The model under review builds one solid part; all positions refer to its coordinate system, in mm. A direction names the side the tool comes from. Give positions to 0.01 mm unless a question says otherwise; leave off trailing zeros. Loops run counter-clockwise (first coordinate to the right, second up) from the corner with the lowest first, then second, coordinate; pieces in that order, holes last. Notation, with made-up numbers: M 12.25,34 L 51.25,34 A24 cw 51.25,45 Z; hole C 72,56.5 d4. An arc over 180 degrees is marked long. Return JSON: item names as keys, results as strings. Group by question number.
```python
from build123d import *

# Parameters (mm, degrees)
LINEAR_AUSTRAGEN1_DEPTH      = 4.035
LINEAR_AUSTRAGEN1_DEPTH_BACK = 4.035


with BuildPart() as part:
    # Skizze1 → Rotation1 (revolve)
    with BuildSketch(Plane.XY, mode=Mode.PRIVATE) as rotation1_sk:
        Polygon((0, 13.2), (3.45, 13.2), (4.35078189, 11.6398), (6, 11.6398), (6.9, 11.220123108), (6.9, -11.742857143), (6.21, -11.742857143), (6.21, -13.7), (4.864, -13.7), (4.864, -18.019), (4.283, -18.6), (3.648, -18.6), (3.648, -8.872), (0, -8.872), align=None)
    revolve(rotation1_sk.sketch.rotate(Axis((0, -18.6, 0), (0, 1, 0)), 270), axis=Axis((0, -18.6, 0), (0, 1, 0)))

    # Skizze2 → Linear austragen1 (cut, two sides: drawn at the far end of the back side and taken through both)
    with BuildSketch(Plane(origin=(0, 11.6398, 0), x_dir=(-1, 0, 0), z_dir=(0, 1, 0)).offset(-LINEAR_AUSTRAGEN1_DEPTH_BACK)):
        Polygon((7.8, -4.5033321), (7.8, 4.5033321), (0, 9.006664199), (-7.8, 4.5033321), (-7.8, -4.5033321), (-0.05, -8.977796686), (-0.05, -6.899335717), (-6, -3.464101615), (-6, 3.464101615), (0, 6.92820323), (6, 3.464101615), (6, -3.464101615), (0, -6.92820323), (0, -9.006664199), align=None)
    extrude(amount=LINEAR_AUSTRAGEN1_DEPTH + LINEAR_AUSTRAGEN1_DEPTH_BACK, mode=Mode.SUBTRACT)

    # Skizze3 → Rotation2 (revolve)
    with BuildSketch(Plane.XY, mode=Mode.PRIVATE) as rotation2_sk:
        Polygon((0, 0), (0, 6.21), (8.832, 6.21), (10.902, 6.25), (18.761, 6.25), (18.761, 5), (21.074, 5), (21.074, 4.166666667), (23.387, 4.166666667), (23.387, 6.25), (25.186, 6.25), (25.7, 4.331725885), (25.7, 3), (7.7, 3), (7.7, 0), align=None)
    revolve(rotation2_sk.sketch.rotate(Axis((25.7, 0, 0), (-1, 0, 0)), 270), axis=Axis((25.7, 0, 0), (-1, 0, 0)))


solid = part.part
```
(1) For faces 1 (the flat face through (3, 7.605, 6)), 2 (the flat face through (3.2, 7.605, -5.4)), 3 (the cylindrical face through (16.57, 0.9, 2.86)), 4 (the flat face through (-6, 10, 0)), list the 3-axis set-ups (+Z, -Z, +X, -X, +Y, -Y) from which the entire face can be reached by the end or side of a thin tool; tool diameter is ignored.
(2) Mouldability with a two-part tool opening along X and no side actions: class faces 5 (the cylindrical face through (1.46, -15.89, 4.64)), 6 (the flat face through (-2, -13.7, -5)), 7 (the cylindrical face through (6.608, 0.273, -6.204)) as released by +X, released by -X, zero draft, split by the parting line, or undercut.
(3) For probe 1 along X at (y, z) = (-14.5, 0); probe 2 along Y at (x, z) = (20, 0); probe 3 along Y at (x, z) = (15, 0), list the stretches that pass through material, from the lowest coordinate up.
(4) Add section C-C (x = 9.5). Write out the cut boundary in (y, z).
(5) For pin 1 (1 mm diameter, centred on y = -8, z = 1.5, fed in from -X); pin 2 (4 mm diameter, centred on x = 6.5, y = 6.5, fed in from -Z); pin 3 (3.5 mm diameter, centred on x = -2, z = 6, fed in from +Y); pin 4 (5 mm diameter, centred on y = 1, z = 0, fed in from +X), all flat-tipped, find the tip position at first contact; note any pin that passes through.
(6) Add section B-B (y = -13). Write out the cut boundary in (x, z).
Verdict:
{
 "1": {"face 1": "+Z, +X, +Y", "face 2": "-Z, +X, +Y", "face 3": "+X", "face 4": "+Z, -Z, -X, +Y"},
 "2": {"face 5": "split by the parting line", "face 6": "zero draft", "face 7": "undercut"},
 "3": {"probe 1": "x = -4.86 to -3.65, 3.65 to 4.86", "probe 2": "y = -5 to -3, 3 to 5", "probe 3": "y = -6.25 to -3, 3 to 6.25"},
 "4": {"outline": "C 0,0 d12.45; hole C 0,0 d6"},
 "5": {"pin 1": "stops at x = -6.83", "pin 2": "stops at z = -5.23", "pin 3": "stops at y = 11.64", "pin 4": "stops at x = 25.7"},
 "6": {"outline": "C 0,0 d12.42; hole C 0,0 d7.3"}
}
